Could you check a few things on this model? Use its own coordinates, in mm. Face numbers are marked on the shaded views. A direction names the side the tool comes from. Round coordinates to 2 decimals unless told otherwise and drop trailing zeros. Loops run counter-clockwise (first coordinate to the right, second up) from the corner with the lowest first, then second, coordinate; pieces in that order, holes last. Notation, with made-up numbers: (34, 29.25) -> (78, 29.25) arc R19 cw to (78, 61.25) -> close; hole circle Ø2 at (-12, 30). An arc over 180 degrees is marked (long way). One line per item, written item: value.
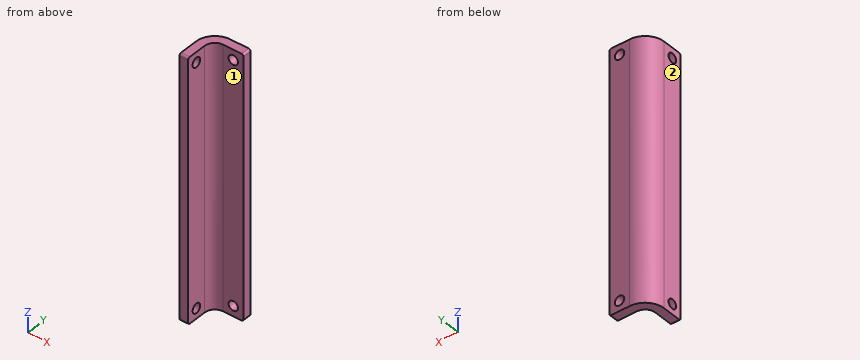
from build123d import *

# Parameters (mm, degrees)
F1_DEPTH = 101.6
F2_R     = 3.96748
F3_R     = 7.38632
F4_R     = 1.8288
F5_DEPTH = 3.41884
F6_R     = 1.8288
F7_DEPTH = 3.41884
F8_R     = 0.762


with BuildPart() as f1:
    # F0 (on Top) → F1 (new body)
    with BuildSketch(Plane.XY):
        Polygon((-3.41884, 0), (0, 0), (0, 11.90498), (11.90498, 11.90498), (11.90498, 15.32382), (-3.41884, 15.32382), align=None)
    extrude(amount=F1_DEPTH)

    # F2
    f2_edges = [f1.edges().sort_by_distance(p)[0] for p in [
        (0, 11.90498, 50.8),
    ]]
    fillet(f2_edges, radius=F2_R)

    # F3
    f3_edges = [f1.edges().sort_by_distance(p)[0] for p in [
        (-3.41884, 15.32382, 50.8),
    ]]
    fillet(f3_edges, radius=F3_R)

    # F4 (on face) → F5 (cut, through all)
    with BuildSketch(Plane(origin=(0, 15.32382, 0), x_dir=(-1, 0, 0), z_dir=(0, 1, 0))):
        with Locations((-7.93623, 97.63125)):
            Circle(F4_R)
        with Locations((-7.93623, 3.96875)):
            Circle(F4_R)
    extrude(amount=-F5_DEPTH, mode=Mode.SUBTRACT)

    # F6 (on face) → F7 (cut, through all)
    with BuildSketch(Plane(origin=(-3.41884, 0, 0), x_dir=(0, -1, 0), z_dir=(-1, 0, 0))):
        with Locations((-3.96875, 97.63125)):
            Circle(F6_R)
        with Locations((-3.96875, 3.96875)):
            Circle(F6_R)
    extrude(amount=-F7_DEPTH, mode=Mode.SUBTRACT)

    # F8
    f8_edges = [f1.edges().sort_by_distance(p)[0] for p in [
        (-1.70942, 0, 101.6),
        (11.90498, 13.6144, 101.6),
        (11.90498, 13.6144, 0),
        (-1.70942, 0, 0),
    ]]
    fillet(f8_edges, radius=F8_R)


solid = f1.part
(1) If we section it at B-B, the plane z = 13.5: Please give me the cut outline in (x, y), then the cut area to 3 significant figures.
Recorded:
outline: (-3.42, 0) -> (0, 0) -> (0, 7.94) arc R3.97 cw to (3.97, 11.9) -> (11.9, 11.9) -> (11.9, 15.32) -> (3.97, 15.32) arc R7.39 ccw to (-3.42, 7.94) -> close
area: 84.8 mm²
(2) If we section it at D-D, the plane y = 10: Please give me the cut outline in (x, z), then the cut area to 3 significant figures.
Recorded:
outline: (-3.13, 0) -> (0.58, 0) -> (0.58, 101.6) -> (-3.13, 101.6) -> close
area: 376 mm²
(3) If I drill on L1, parallel to Z at x = 7, y = 13; L2, parallel to Z at x = 9.25, y = 12; L3, parallel to Y at x = 5, z = 38, over which ranges is the centre line in solid material (lowest first)?
Recorded:
L1: 0 to 2.4, 5.54 to 96.06, 99.2 to 101.6
L2: 0 to 2.7, 5.24 to 96.36, 98.9 to 101.6
L3: 11.9 to 15.32
(4) For the marked faces 1 and 2, which set-ups out of +Z, -Z, +X, -X, +Y, -Y let a thin tool reach every point of the face, with its end or its side?
Recorded:
face 1: +Z, -Z, +X, -Y
face 2: +Z, -Z, -X, +Y, -Y
(5) If we section it at A-A, the plane y = 4: Please give me the cut outline in (x, z).
Recorded:
outline: (-3.42, 0) -> (0, 0) -> (0, 2.14) -> (-3.42, 2.14) -> close; (-3.42, 5.8) -> (0, 5.8) -> (0, 95.8) -> (-3.42, 95.8) -> close; (-3.42, 99.46) -> (0, 99.46) -> (0, 101.6) -> (-3.42, 101.6) -> close
(6) If we section it at C-C, the plane x = 1: Please give me the cut outline in (y, z).
Recorded:
outline: (10.57, 0) -> (14.7, 0) -> (14.7, 101.6) -> (10.57, 101.6) -> close
(7) I'm going to push flat-ended pins straight in: pin 1 Ø2 at (y, z) = (10.5, 30.5) entering from +X; pin 2 Ø4 at (y, z) = (3.97, 3.97) entering from +X; pin 3 Ø3.5 at (x, z) = (7.94, 3.97) entering from -Y; pin 4 Ø8 at (x, z) = (2.5, 66.5) entering from +Y. Where does each tip first touch, or does it pass through?
Recorded:
pin 1: x = 2.22
pin 2: x = 0
pin 3: through
pin 4: y = 15.32
